Autodesk Inventor part; units mm, degrees
ref_plane "YZ Plane" through (0, 0, 0) normal (1, 0, 0) x (0, 1, 0)
ref_plane "XZ Plane" through (0, 0, 0) normal (0, 1, 0) x (-1, 0, 0)
ref_plane "XY Plane" through (0, 0, 0) normal (0, 0, 1) x (1, 0, 0)
sketch "Sketch1" plane through (0, 0, 0) normal (0, 1, 0) x (-1, 0, 0)
  line L0 (0, 0) -> (-101.6, 0)
  line L1 (-101.6, 0) -> (-101.6, -133.35)
  line L2 (-101.6, -133.35) -> (0, -133.35)
  line L3 (0, -133.35) -> (0, 0)
  dimension "d0" = 101.6
  dimension "d1" = 133.35
extrude "Extrusion1" add sketch "Sketch1" along normal blind 5.08
sketch "Sketch2" plane through (0, 5.08, 0) normal (0, 1, 0) x (1, 0, 0)
  line L0 (101.6, 133.35) -> (0, 133.35)
  line L1 (50.8, 133.35) -> (50.8, 114.3)
  line L2 (50.8, 114.3) -> (22.225, 114.3)
  line L3 (22.225, 114.3) -> (22.225, 85.725)
  line L4 (22.225, 85.725) -> (50.8, 85.725)
  line L5 (50.8, 85.725) -> (50.8, 114.3)
  point P0 (0, 0)
  dimension "d4" = 19.05
  dimension "d5" = 28.575
  dimension "d6" = 28.575
extrude "Extrusion2" cut sketch "Sketch2" against normal blind 25.4
properties part number "HalfofTop"
Check sheet for the modelled part. Datum: model origin and axes. Units: mm. A direction names the side the tool comes from. Give positions to 0.01 mm unless a question says otherwise; leave off trailing zeros. Order: outer loops, then holes, each group sorted by start corner. A loop starts at its lowest first (then second) coordinate and runs counter-clockwise, first axis right, second up. Notation, with made-up numbers: M 48.25,52.25 L 106.25,52.25 A6 ccw 106.25,63.25 Z; hole C 54,77 d8. An arc over 180 degrees is marked long. Answer in a Markdown table with one row per item. Add a question column.
Q1. Sectioned sample at C-C, the plane y = 4.25. Record the boundary of the cut face in (x, z) (3 decimals), and give its area (3 significant figures).
Q2. Release check for a two-part mould opening along X. For faces 3 (the flat face through (0, 3, -68)), 4 (the flat face through (37, 3, -114.3)), 5 (the flat face through (52, 3, -133.35)) record: released by +X, released by -X, zero draft, split by the parting line, or undercut.
Q3. Sectioned sample at A-A, the plane x = 32. Record the boundary of the cut face in (y, z) (3 decimals).
Q4. Thickness scan on L1, parallel to X at y = 1.1, z = -112 (3 decimals); L2, parallel to Z at x = 25.5, y = 3.45 (3 decimals). Record the ranges inside material, lowest first.
Q5. Sectioned sample at B-B, the plane z = -100. Record the boundary of the cut face in (x, y) (3 decimals).
Q6. Access from +Z, -Z, +X, -X, +Y, -Y to the whole of each face (thin tool, end or side, straight path). Record for faces 1 (the flat face through (52, 0, -66)), 2 (the flat face through (50.8, 3, -100)).
Verdict:
| question | item | result |
|---|---|---|
| 1 | outline | M 0,-133.35 L 101.6,-133.35 L 101.6,0 L 0,0 Z; hole M 22.225,-114.3 L 50.8,-114.3 L 50.8,-85.725 L 22.225,-85.725 Z |
| 1 | area | 12,700 mm² |
| 2 | face 3 | released by -X |
| 2 | face 4 | undercut |
| 2 | face 5 | zero draft |
| 3 | outline | M 0,-133.35 L 5.08,-133.35 L 5.08,-114.3 L 0,-114.3 Z; M 0,-85.725 L 5.08,-85.725 L 5.08,0 L 0,0 Z |
| 4 | L1 | 0 to 22.225, 50.8 to 101.6 |
| 4 | L2 | -133.35 to -114.3, -85.725 to 0 |
| 5 | outline | M 0,0 L 22.225,0 L 22.225,5.08 L 0,5.08 Z; M 50.8,0 L 101.6,0 L 101.6,5.08 L 50.8,5.08 Z |
| 6 | face 1 | +Z, -Z, +X, -X, -Y |
| 6 | face 2 | +Y, -Y |
